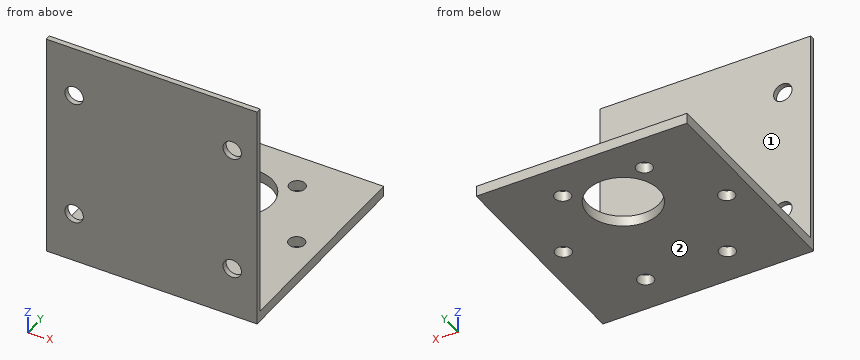
from build123d import *

# Parameters (mm, degrees)
SKETCH1_W           = 40
SKETCH1_H           = 43
SKETCH1_R           = 1.75
BOSS_EXTRUDE1_DEPTH = 1
SKETCH4_W           = 40
SKETCH4_H           = 2
BOSS_EXTRUDE2_DEPTH = 40
SKETCH5_R           = 6.75
CUT_EXTRUDE5_DEPTH  = 34
SKETCH8_R           = 1.5
CUT_EXTRUDE6_DEPTH  = 10


with BuildPart() as part:
    # Sketch1 → Boss-Extrude1 (new body)
    with BuildSketch(Plane(origin=(0, 0, 0), x_dir=(1, 0, 0), z_dir=(0, 1, 0))):
        Rectangle(SKETCH1_W, SKETCH1_H)
        with Locations(Location((-14.715053003, 12, 0), (0, 0, 270))):
            Circle(SKETCH1_R, mode=Mode.SUBTRACT)
        with Locations(Location((15.284946997, 12, 0), (0, 0, 270))):
            Circle(SKETCH1_R, mode=Mode.SUBTRACT)
        with Locations(Location((-14.715053003, -12, 0), (0, 0, 270))):
            Circle(SKETCH1_R, mode=Mode.SUBTRACT)
        with Locations(Location((15.284946997, -12, 0), (0, 0, 270))):
            Circle(SKETCH1_R, mode=Mode.SUBTRACT)
    extrude(amount=-BOSS_EXTRUDE1_DEPTH)

    # Sketch4 → Boss-Extrude2 (add)
    with BuildSketch(Plane(origin=(0, 0, 0), x_dir=(1, 0, 0), z_dir=(0, 1, 0))):
        with Locations((0, 20.5)):
            Rectangle(SKETCH4_W, SKETCH4_H)
    extrude(amount=BOSS_EXTRUDE2_DEPTH)

    # Sketch5 → Cut-Extrude5 (cut)
    with BuildSketch(Plane.XY.offset(-19.5)):
        with Locations((0, 26.5)):
            Circle(SKETCH5_R)
    extrude(amount=-CUT_EXTRUDE5_DEPTH, mode=Mode.SUBTRACT)

    # Sketch8 → Cut-Extrude6 (cut)
    with BuildSketch(Plane.XY.offset(-19.5)):
        with Locations((-15.5, 19.5)):
            Circle(SKETCH8_R)
        with Locations((-7.75, 32.923393759)):
            Circle(SKETCH8_R)
        with Locations((7.75, 32.923393759)):
            Circle(SKETCH8_R)
        with Locations((15.5, 19.5)):
            Circle(SKETCH8_R)
        with Locations((7.75, 6.076606241)):
            Circle(SKETCH8_R)
        with Locations((-7.75, 6.076606241)):
            Circle(SKETCH8_R)
    extrude(amount=-CUT_EXTRUDE6_DEPTH, mode=Mode.SUBTRACT)


solid = part.part
Build history of the part. All positions in model axes, mm. Face numbers are marked on the shaded views. A direction names the side the tool comes from. Round coordinates to 2 decimals unless told otherwise and drop trailing zeros. Write each loop counter-clockwise with the first axis right and the second up, starting at its lowest first coordinate (ties: lowest second). Pieces come first, ordered by that corner, then holes. Notation, with made-up numbers: M -12.75,-32 L 27.25,-32 A35 ccw 27.25,0 Z; hole C -8,18.25 d3. An arc over 180 degrees is marked long. Answer as a JSON object with one key per item and string values. Group by question number.
(1) Cut at C-C (z = -11). Give the cut face in (x, y), and give its area (3 significant figures).
(2) Which spindle directions (+Z, -Z, +X, -X, +Y, -Y) get a long thin tool onto all of the face, cutting with end or side? Do the marked faces 1 and 2. Say none if no direction does.
(3) Flat gauge pins, fed straight in: pin 1 (8 mm diameter, centred on x = 0, y = 26.5, fed in from -Z); pin 2 (4 mm diameter, centred on x = -7.75, y = 6.08, fed in from +Z); pin 3 (5 mm diameter, centred on x = 12.5, z = -3.5, fed in from +Y). Where does each tip first touch, or does it go through?
(4) Drill centre lines: L1, parallel to Y at x = 7.75, z = -20.55; L2, parallel to Z at x = -12.5, y = 31; L3, parallel to Y at x = -5.5, z = 13. Where is each one in solid material? Low to high.
(5) Cut at A-A (y = 26.5). Give the cut face in (x, z).
(6) Cut at D-D (x = 1). Give the cut face in (y, z), and give its area (3 significant figures).
(7) Cut at B-B (x = -8.5). Give the cut face in (y, z).
Responses:
{
 "1": {"outline": "M -20,-1 L -16.15,-1 L -16.15,0 L -20,0 Z; M -13.28,-1 L 13.85,-1 L 13.85,0 L -13.28,0 Z; M 16.72,-1 L 20,-1 L 20,0 L 16.72,0 Z", "area": "34.3 mm2"},
 "2": {"face 1": "+Z, +X, -X, +Y", "face 2": "-Z, +X, -X, +Y, -Y"},
 "3": {"pin 1": "passes through", "pin 2": "stops at z = -19.5", "pin 3": "stops at y = 0"},
 "4": {"L1": "y = -1 to 4.58, 7.58 to 31.42, 34.42 to 40", "L2": "z = -21.5 to -19.5", "L3": "y = -1 to 0"},
 "5": {"outline": "M -20,-21.5 L -6.75,-21.5 L -6.75,-19.5 L -20,-19.5 Z; M 6.75,-21.5 L 20,-21.5 L 20,-19.5 L 6.75,-19.5 Z"},
 "6": {"outline": "M -1,-21.5 L 19.82,-21.5 L 19.82,-19.5 L 0,-19.5 L 0,21.5 L -1,21.5 Z; M 33.18,-21.5 L 40,-21.5 L 40,-19.5 L 33.18,-19.5 Z", "area": "96.3 mm2"},
 "7": {"outline": "M -1,-21.5 L 4.78,-21.5 L 4.78,-19.5 L 0,-19.5 L 0,21.5 L -1,21.5 Z; M 7.38,-21.5 L 31.62,-21.5 L 31.62,-19.5 L 7.38,-19.5 Z; M 34.22,-21.5 L 40,-21.5 L 40,-19.5 L 34.22,-19.5 Z"}
}
